Here's how the part is built. I have some questions about the finished solid (model axes, mm). A direction names the side the tool comes from. Coordinates: 2 decimals unless noted, no trailing zeros. Order: outer loops, then holes, each group sorted by start corner. A loop starts at its lowest first (then second) coordinate and runs counter-clockwise, first axis right, second up. Notation, with made-up numbers: (2, -26) - (42, -26) arc R21 cw to (42, 4) - close; hole circle Ø1 at (66, -30). An arc over 180 degrees is marked (long way). Answer in a Markdown table with one row per item. Add a question column.
Item 1: I want a section at A-A (y = 1.5). Please give me the cut outline in (x, z).
Item 2: If I drill on line 1 along X through (y, z) = (9.35, 0); line 2 along X through (y, z) = (4.75, -0.25); line 3 along Y through (x, z) = (-19, -2.5), over which ranges is the centre line in solid material (lowest first)? Write a range as from..to.
Item 3: I want a section at D-D (x = 0). Please give me the cut outline in (y, z).
Item 4: Will these pins go through, and if not, where does the flat tip stop? pin 1 Ø2.5 at (y, z) = (3, -0.5) entering from +X; pin 2 Ø3.5 at (y, z) = (3, -1) entering from -X; pin 3 Ø5 at (x, z) = (-0.5, 3.5) entering from -Y; pin 4 Ø3 at (y, z) = (5.5, 7.5) entering from -X.
Item 5: On a 3-axis mill with a long thin cutter (end or side, diameter ignored), from which of +Z, -Z, +X, -X, +Y, -Y can I reach the whole of each face in a straight line? I mean faces 4 (the flat face through (-7, 5.2, 0.1)), 5 (the flat face through (-25.5, 2, 0)), 6 (the flat face through (0, 4, 7)), 7 (the flat face through (-24, 2, -2.5)). Say none if no direction works.
Item 6: I want a section at B-B (x = -18.5). Please give me the cut outline in (y, z).
Item 7: I want a section at C-C (z = -9). Please give me the cut outline in (x, y).
Item 8: Thinking about a two-plate mould opening in X: for faces 1 (the cylindrical face through (24.07, 3.01, -4.55)), 2 (the flat face through (0, 4, -7)), 3 (the cylindrical face through (21.95, 3.01, -4.57)), which applies, +X half, -X half, draft (parallel to the pull), parting line (faces both ways), or undercut?
```python
from build123d import *

# Parameters (mm, degrees)
BOSS_EXTRUDE1_DEPTH = 1
SKETCH2_W           = 14
SKETCH2_H           = 14
BOSS_EXTRUDE2_DEPTH = 7
SKETCH3_R           = 4
BOSS_EXTRUDE3_DEPTH = 1.5
BOSS_EXTRUDE4_DEPTH = 4
SKETCH6_R           = 1
CUT_EXTRUDE1_DEPTH  = 1
CUT_EXTRUDE2_REACH  = 32.191
SKETCH7_R           = 1
SKETCH8_R           = 3.5
BOSS_EXTRUDE5_DEPTH = 4
SKETCH9_W           = 4
SKETCH9_H           = 4
BOSS_EXTRUDE6_DEPTH = 3
SKETCH11_W          = 4
SKETCH11_H          = 11
BOSS_EXTRUDE7_DEPTH = 1
SKETCH12_W          = 3
SKETCH12_H          = 10
BOSS_EXTRUDE8_DEPTH = 2
FILLET1_R           = 1.5


with BuildPart() as part:
    # Sketch1 → Boss-Extrude1 (new body)
    with BuildSketch(Plane(origin=(0, 0, 0), x_dir=(1, 0, 0), z_dir=(0, 1, 0))):
        Polygon((-22, -10.5), (22, -10.5), (27, -5.5), (27, 5.5), (22, 10.5), (-22, 10.5), (-27, 5.5), (-27, -5.5), align=None)
    extrude(amount=BOSS_EXTRUDE1_DEPTH)

    # Sketch2 → Boss-Extrude2 (add)
    with BuildSketch(Plane(origin=(0, 1, 0), x_dir=(1, 0, 0), z_dir=(0, 1, 0))):
        Rectangle(SKETCH2_W, SKETCH2_H)
    extrude(amount=BOSS_EXTRUDE2_DEPTH)

    # Sketch3 → Boss-Extrude3 (add)
    with BuildSketch(Plane(origin=(0, 8, 0), x_dir=(1, 0, 0), z_dir=(0, 1, 0))):
        with Locations(Location((0, 0, 0), (0, 0, 270))):
            Circle(SKETCH3_R)
    extrude(amount=BOSS_EXTRUDE3_DEPTH)

    # Sketch4 → Boss-Extrude4 (add)
    with BuildSketch(Plane(origin=(0, 1, 0), x_dir=(1, 0, 0), z_dir=(0, 1, 0))):
        with BuildLine():
            ThreePointArc((7, -3), (9.121320344, -2.121320344), (10, 0))
            ThreePointArc((10, 0), (9.121320344, 2.121320344), (7, 3))
            Line((7, 3), (7, -3))
        make_face()
        with BuildLine():
            Line((7, -3), (7, 3))
            ThreePointArc((7, 3), (4, 0), (7, -3))
        make_face()
        with BuildLine():
            ThreePointArc((-7, -3), (-4.878679656, -2.121320344), (-4, 0))
            ThreePointArc((-4, 0), (-4.878679656, 2.121320344), (-7, 3))
            Line((-7, 3), (-7, -3))
        make_face()
        with BuildLine():
            Line((-7, -3), (-7, 3))
            ThreePointArc((-7, 3), (-10, 0), (-7, -3))
        make_face()
    extrude(amount=BOSS_EXTRUDE4_DEPTH)

    # Sketch6 → Cut-Extrude1 (cut)
    with BuildSketch(Plane(origin=(0, 9.5, 0), x_dir=(1, 0, 0), z_dir=(0, 1, 0))):
        with Locations(Location((0, 0, 0), (0, 0, 270))):
            Circle(SKETCH6_R)
    extrude(amount=-CUT_EXTRUDE1_DEPTH, mode=Mode.SUBTRACT)

    # Sketch7 → Cut-Extrude2 (cut, up to next)
    with BuildSketch(Plane(origin=(0, 1, 0), x_dir=(1, 0, 0), z_dir=(0, 1, 0)), mode=Mode.PRIVATE) as cut_extrude2_sk1:
        with Locations(Location((-18.5, 9, 0), (0, 0, 270))):
            Circle(SKETCH7_R)
    cut_extrude2_tool1 = extrude(cut_extrude2_sk1.sketch, amount=-CUT_EXTRUDE2_REACH, mode=Mode.PRIVATE) & part.part
    # Sketch7 → Cut-Extrude2 (cut, up to next)
    with BuildSketch(Plane(origin=(0, 1, 0), x_dir=(1, 0, 0), z_dir=(0, 1, 0)), mode=Mode.PRIVATE) as cut_extrude2_sk2:
        with Locations(Location((21, -9, 0), (0, 0, 270))):
            Circle(SKETCH7_R)
    cut_extrude2_tool2 = extrude(cut_extrude2_sk2.sketch, amount=-CUT_EXTRUDE2_REACH, mode=Mode.PRIVATE) & part.part
    add(cut_extrude2_tool1.solids().sort_by_distance((-18.5, 1, -9))[0], mode=Mode.SUBTRACT)
    add(cut_extrude2_tool2.solids().sort_by_distance((21, 1, 9))[0], mode=Mode.SUBTRACT)

    # Sketch8 → Boss-Extrude5 (add)
    with BuildSketch(Plane(origin=(0, 1, 0), x_dir=(1, 0, 0), z_dir=(0, 1, 0))):
        with Locations(Location((-17, 0, 0), (0, 0, 90))):
            Circle(SKETCH8_R)
    extrude(amount=BOSS_EXTRUDE5_DEPTH)

    # Sketch9 → Boss-Extrude6 (add)
    with BuildSketch(Plane(origin=(0, 1, 0), x_dir=(1, 0, 0), z_dir=(0, 1, 0))):
        with Locations((-23.5, 0.5)):
            Rectangle(SKETCH9_W, SKETCH9_H)
    extrude(amount=BOSS_EXTRUDE6_DEPTH)

    # Sketch11 → Boss-Extrude7 (add)
    with BuildSketch(Plane(origin=(0, 1, 0), x_dir=(1, 0, 0), z_dir=(0, 1, 0))):
        with Locations((23, 0)):
            Rectangle(SKETCH11_W, SKETCH11_H)
    extrude(amount=BOSS_EXTRUDE7_DEPTH)

    # Sketch12 → Boss-Extrude8 (add)
    with BuildSketch(Plane(origin=(0, 2, 0), x_dir=(1, 0, 0), z_dir=(0, 1, 0))):
        with Locations((23, 0)):
            Rectangle(SKETCH12_W, SKETCH12_H)
    extrude(amount=BOSS_EXTRUDE8_DEPTH)

    # Fillet1
    fillet1_edges = [part.edges().sort_by_distance(p)[0] for p in [
        (24.5, 3, -5),
        (21.5, 3, -5),
        (21.5, 3, 5),
        (24.5, 3, 5),
    ]]
    fillet(fillet1_edges, radius=FILLET1_R - 0.0001)  # a hair under: the kernel refuses the full size


solid = part.part
```
Values follow:
| question | item | result |
|---|---|---|
| 1 | outline | (-25.5, -2.5) - (-21.5, -2.5) - (-21.5, 1.5) - (-25.5, 1.5) - close; circle Ø7 at (-17, 0); (-7, -7) - (7, -7) - (7, -3) arc R3 ccw to (7, 3) - (7, 7) - (-7, 7) - (-7, 3) arc R3 ccw to (-7, -3) - close; (21, -5.5) - (25, -5.5) - (25, 5.5) - (21, 5.5) - close |
| 2 | line 1 | x = -4..-1, 1..4 |
| 2 | line 2 | x = -20.49..-13.51, -9.99..9.99 |
| 2 | line 3 | y = 0..5 |
| 3 | outline | (0, -10.5) - (1, -10.5) - (1, -7) - (8, -7) - (8, -4) - (9.5, -4) - (9.5, -1) - (8.5, -1) - (8.5, 1) - (9.5, 1) - (9.5, 4) - (8, 4) - (8, 7) - (1, 7) - (1, 10.5) - (0, 10.5) - close |
| 4 | pin 1 | stops at x = 25 |
| 4 | pin 2 | stops at x = -25.5 |
| 4 | pin 3 | stops at y = 0 |
| 4 | pin 4 | stops at x = -7 |
| 5 | face 4 | +Y |
| 5 | face 5 | +Z, -Z, -X, +Y |
| 5 | face 6 | +Z, +X, -X, +Y |
| 5 | face 7 | -Z, -X, +Y |
| 6 | outline | (0, -10.5) - (1, -10.5) - (1, -10) - (0, -10) - close; (0, -8) - (1, -8) - (1, -3.16) - (5, -3.16) - (5, 3.16) - (1, 3.16) - (1, 10.5) - (0, 10.5) - close |
| 7 | outline | (-23.5, 0) - (-19.5, 0) - (-19.5, 1) - (-23.5, 1) - close; (-17.5, 0) - (23.5, 0) - (23.5, 1) - (-17.5, 1) - close |
| 8 | face 1 | +X half |
| 8 | face 2 | draft |
| 8 | face 3 | undercut |
